from build123d import *

# Parameters (mm, degrees)
SKETCH1_R                 = 2.7503
SKETCH1_R_2               = 1.575
SKETCH1_W                 = 50
SKETCH1_H                 = 50
BOSS_EXTRUDE1_DEPTH       = 1.524
SKETCH2_W                 = 15
SKETCH2_H                 = 2.5
SKETCH2_W_2               = 2.5
SKETCH2_H_2               = 15
BOSS_EXTRUDE2_DEPTH       = 12.476
SKETCH3_R                 = 2.125
CUT_EXTRUDE1_DEPTH        = 1
CUT_EXTRUDE1_DEPTH_BACK   = 101
SKETCH4_R                 = 2.125
CUT_EXTRUDE2_DEPTH        = 1
CUT_EXTRUDE2_DEPTH_BACK   = 101
SKETCH5_W                 = 60
SKETCH5_H                 = 1
SKETCH5_W_2               = 1
SKETCH5_H_2               = 60
CUT_EXTRUDE3_DEPTH        = 1
CUT_EXTRUDE3_DEPTH_BACK   = 15
SKETCH6_R                 = 4.445
BOSS_EXTRUDE3_DEPTH       = 15
F_5_40_TAPPED_HOLE1_D     = 2.5781
F_5_40_TAPPED_HOLE1_DEPTH = 15
F_5_40_TAPPED_HOLE1_TIP   = 0.774539381


with BuildPart() as part:
    # Sketch1 → Boss-Extrude1 (new body)
    with BuildSketch(Plane(origin=(0, 0, 0), x_dir=(1, 0, 0), z_dir=(0, 1, 0))):
        Polygon((41.364, 50), (-41.364, 50), (-41.364, 48.73), (-47.079, 48.73), (-48.73, 47.079), (-48.73, 41.364), (-50, 41.364), (-50, -41.364), (-48.73, -41.364), (-48.73, -47.079), (-47.079, -48.73), (-41.364, -48.73), (-41.364, -50), (41.364, -50), (41.364, -48.73), (47.079, -48.73), (48.73, -47.079), (48.73, -41.364), (50, -41.364), (50, 41.364), (48.73, 41.364), (48.73, 47.079), (47.079, 48.73), (41.364, 48.73), align=None)
        with Locations((-45.2, -45.2)):
            Circle(SKETCH1_R, mode=Mode.SUBTRACT)
        with Locations((-24.7, -46.8)):
            Circle(SKETCH1_R_2, mode=Mode.SUBTRACT)
        with Locations((24.7, -46.8)):
            Circle(SKETCH1_R_2, mode=Mode.SUBTRACT)
        with Locations((45.2, -45.2)):
            Circle(SKETCH1_R, mode=Mode.SUBTRACT)
        Rectangle(SKETCH1_W, SKETCH1_H, mode=Mode.SUBTRACT)
        with Locations((-45.2, 45.2)):
            Circle(SKETCH1_R, mode=Mode.SUBTRACT)
        with Locations((-24.7, 46.8)):
            Circle(SKETCH1_R_2, mode=Mode.SUBTRACT)
        with BuildLine():
            ThreePointArc((26.275, 46.8), (24.7, 45.225), (23.125, 46.8))
            ThreePointArc((23.125, 46.8), (24.7, 48.375), (26.275, 46.8))
        make_face(mode=Mode.SUBTRACT)
        with Locations((45.2, 45.2)):
            Circle(SKETCH1_R, mode=Mode.SUBTRACT)
    extrude(amount=BOSS_EXTRUDE1_DEPTH)

    # Sketch2 → Boss-Extrude2 (add)
    with BuildSketch(Plane(origin=(0, 1.524, 0), x_dir=(1, 0, 0), z_dir=(0, 1, 0))):
        with Locations((0, 48.75)):
            Rectangle(SKETCH2_W, SKETCH2_H)
        with Locations((48.75, 0)):
            Rectangle(SKETCH2_W_2, SKETCH2_H_2)
        with Locations((0, -48.75)):
            Rectangle(SKETCH2_W, SKETCH2_H)
        with Locations((-48.75, 0)):
            Rectangle(SKETCH2_W_2, SKETCH2_H_2)
    extrude(amount=BOSS_EXTRUDE2_DEPTH)

    # Sketch3 → Cut-Extrude1 (cut, two sides)
    with BuildSketch(Plane.XY.offset(50)) as cut_extrude1_sk:
        with BuildLine():
            ThreePointArc((0, 14), (5.303300859, 11.803300859), (7.5, 6.5))
            Line((7.5, 6.5), (7.5, 14))
            Line((7.5, 14), (0, 14))
        make_face()
        with BuildLine():
            ThreePointArc((-7.5, 6.5), (-5.303300859, 11.803300859), (0, 14))
            Line((0, 14), (-7.5, 14))
            Line((-7.5, 14), (-7.5, 6.5))
        make_face()
        with Locations((0, 6.5)):
            Circle(SKETCH3_R)
    extrude(amount=CUT_EXTRUDE1_DEPTH, mode=Mode.SUBTRACT)
    extrude(cut_extrude1_sk.sketch, amount=-CUT_EXTRUDE1_DEPTH_BACK, mode=Mode.SUBTRACT)

    # Sketch4 → Cut-Extrude2 (cut, two sides)
    with BuildSketch(Plane.ZY.offset(50)) as cut_extrude2_sk:
        with Locations((0, 6.5)):
            Circle(SKETCH4_R)
        with BuildLine():
            ThreePointArc((0, 14), (5.303300859, 11.803300859), (7.5, 6.5))
            Line((7.5, 6.5), (7.5, 14))
            Line((7.5, 14), (0, 14))
        make_face()
        with BuildLine():
            ThreePointArc((-7.5, 6.5), (-5.303300859, 11.803300859), (0, 14))
            Line((0, 14), (-7.5, 14))
            Line((-7.5, 14), (-7.5, 6.5))
        make_face()
    extrude(amount=CUT_EXTRUDE2_DEPTH, mode=Mode.SUBTRACT)
    extrude(cut_extrude2_sk.sketch, amount=-CUT_EXTRUDE2_DEPTH_BACK, mode=Mode.SUBTRACT)

    # Sketch5 → Cut-Extrude3 (cut, two sides)
    with BuildSketch(Plane.XZ) as cut_extrude3_sk:
        with Locations((0, -49.5)):
            Rectangle(SKETCH5_W, SKETCH5_H)
        with Locations((-49.5, 0)):
            Rectangle(SKETCH5_W_2, SKETCH5_H_2)
        with Locations((0, 49.5)):
            Rectangle(SKETCH5_W, SKETCH5_H)
        with Locations((49.5, 0)):
            Rectangle(SKETCH5_W_2, SKETCH5_H_2)
    extrude(amount=CUT_EXTRUDE3_DEPTH, mode=Mode.SUBTRACT)
    extrude(cut_extrude3_sk.sketch, amount=-CUT_EXTRUDE3_DEPTH_BACK, mode=Mode.SUBTRACT)

    # Sketch6 → Boss-Extrude3 (add)
    with BuildSketch(Plane(origin=(0, 1.524, 0), x_dir=(1, 0, 0), z_dir=(0, 1, 0))):
        with Locations((30, 30)):
            Circle(SKETCH6_R)
        with Locations((30, -30)):
            Circle(SKETCH6_R)
        with Locations((-30, -30)):
            Circle(SKETCH6_R)
        with Locations((-30, 30)):
            Circle(SKETCH6_R)
    extrude(amount=BOSS_EXTRUDE3_DEPTH)

    # #5-40 Tapped Hole1
    with Locations(Plane(origin=(0, 16.524, 0), x_dir=(1, 0, 0), z_dir=(0, 1, 0))):
        with Locations((-17.222965343, 16.834933913), (-30, 30), (-30, -30), (30, -30), (30, 30)):
            Hole(F_5_40_TAPPED_HOLE1_D / 2, depth=F_5_40_TAPPED_HOLE1_DEPTH)
            with Locations((0, 0, -(F_5_40_TAPPED_HOLE1_DEPTH + F_5_40_TAPPED_HOLE1_TIP / 2))):  # 118° drill point
                Cone(0, F_5_40_TAPPED_HOLE1_D / 2, F_5_40_TAPPED_HOLE1_TIP, mode=Mode.SUBTRACT)


solid = part.part
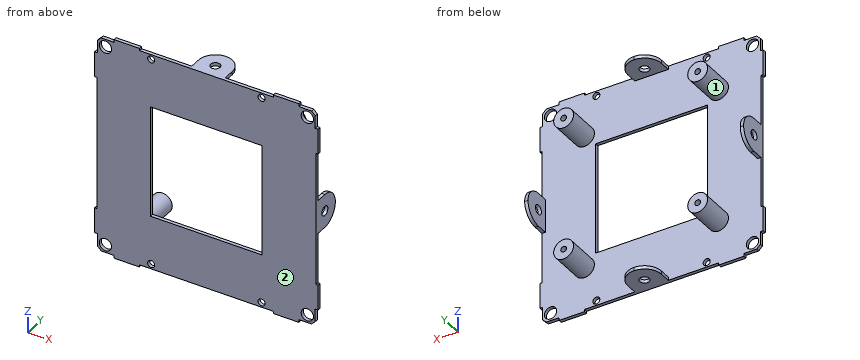
Source: CAD feature listing. Evaluate the final solid. Frame: model axes, mm. Face numbers are marked on the shaded views. Round coordinates to 2 decimals unless told otherwise and drop trailing zeros. Loops run counter-clockwise (first coordinate to the right, second up) from the corner with the lowest first, then second, coordinate; pieces in that order, holes last.
Q1. Section A-A, the plane z = 15.5. Return loops of the section in (x, y).
Q2. Ray query, line 1 (Z direction, x = 30, y = 8) (3 decimals); line 2 (Z direction, x = 45.2, y = 1). Return the intervals inside material, ascending.
Q3. Mould query, pull axis Z, two halves, no side actions, for the marked faces 1 and 2. Classes: pulls with the +Z half, pulls with the -Z half, needs draft (parallel to the pull), parting line crosses it, or undercut.
Q4. First-contact query: P1, Ø0.8, axis at x = 48, y = 3.5, coming from the -Z side; P2, Ø0.8, axis at y = 1, z = -44.5, coming from the +X side; P3, Ø3.5, axis at y = 7, z = 3, coming from the +X side. Flat tips, straight axial feed; report the tip coordinate or a pass-through.
Q5. Section C-C, the plane z = -39. Return loops of the section in (x, y), plus the area to 3 significant figures.
Q6. Section B-B, the plane x = 13. Return loops of the section in (y, z), plus the area to 3 significant figures.
Solutions:
1. outline: (-49, 0) - (-25, 0) - (-25, 1.52) - (-49, 1.52) - close; (25, 0) - (49, 0) - (49, 1.52) - (25, 1.52) - close
2. line 1: z = -34.445 to -31.289, -28.711 to -25.555, 25.555 to 28.711, 31.289 to 34.445
2. line 2: z = -48.73 to -47.95, -42.45 to 42.45, 47.95 to 48.73
3. face 1: undercut
3. face 2: needs draft
4. P1: stops at z = -7.5
4. P2: stops at x = 48.73
4. P3: stops at x = 49
5. outline: (-50, 0) - (50, 0) - (50, 1.52) - (-50, 1.52) - close
5. area: 152 mm2
6. outline: (0, -49) - (1.52, -49) - (1.52, -25) - (0, -25) - close; (0, 25) - (1.52, 25) - (1.52, 49) - (0, 49) - close
6. area: 73.2 mm2
